```python
from build123d import *

# Parameters (mm, degrees)
BOSS_EXTRUDE1_DEPTH = 7.5
SKETCH2_R           = 6.1
BOSS_EXTRUDE2_DEPTH = 2.3
SKETCH3_R           = 7.625
BOSS_EXTRUDE3_DEPTH = 1.3
CUT_EXTRUDE1_DEPTH  = 12.1
CUT_EXTRUDE2_REACH  = 15.91
SKETCH5_R           = 1.5


with BuildPart() as part:
    # Sketch1 → Boss-Extrude1 (new body)
    with BuildSketch(Plane(origin=(0, 0, 0), x_dir=(1, 0, 0), z_dir=(0, 1, 0))):
        Polygon((7.257292884, 0), (3.628646442, 6.285), (-3.628646442, 6.285), (-7.257292884, 0), (-3.628646442, -6.285), (3.628646442, -6.285), align=None)
    extrude(amount=BOSS_EXTRUDE1_DEPTH)

    # Sketch2 → Boss-Extrude2 (add)
    with BuildSketch(Plane(origin=(0, 7.5, 0), x_dir=(1, 0, 0), z_dir=(0, 1, 0))):
        Circle(SKETCH2_R)
    extrude(amount=BOSS_EXTRUDE2_DEPTH)

    # Sketch3 → Boss-Extrude3 (add)
    with BuildSketch(Plane.XZ):
        Circle(SKETCH3_R)
    extrude(amount=BOSS_EXTRUDE3_DEPTH)

    # Sketch4 → Cut-Extrude1 (cut, through all)
    with BuildSketch(Plane(origin=(0, 9.8, 0), x_dir=(1, 0, 0), z_dir=(0, 1, 0))):
        with BuildLine():
            Line((-1.12, -0.997797575), (1.12, -0.997797575))
            ThreePointArc((1.12, -0.997797575), (0, 1.5), (-1.12, -0.997797575))
        make_face()
    extrude(amount=-CUT_EXTRUDE1_DEPTH, mode=Mode.SUBTRACT)

    # Sketch5 → Cut-Extrude2 (cut, up to next)
    with BuildSketch(Plane.XY.offset(6.285), mode=Mode.PRIVATE) as cut_extrude2_sk1:
        with Locations((0, 3.75)):
            Circle(SKETCH5_R)
    cut_extrude2_tool1 = extrude(cut_extrude2_sk1.sketch, amount=-CUT_EXTRUDE2_REACH, mode=Mode.PRIVATE) & part.part
    add(cut_extrude2_tool1.solids().sort_by_distance((0, 3.75, 6.285))[0], mode=Mode.SUBTRACT)


solid = part.part
```
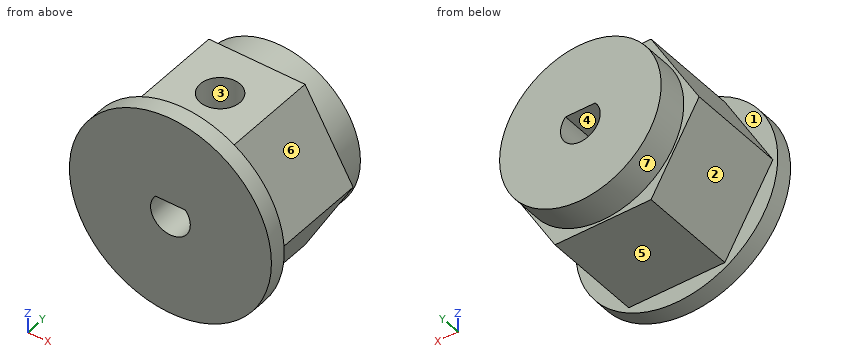
Check sheet for the modelled part. Datum: model origin and axes. Units: mm. Face numbers are marked on the shaded views. A direction names the side the tool comes from. Coordinates: 2 decimals unless noted, no trailing zeros. Order: outer loops, then holes, each group sorted by start corner. A loop starts at its lowest first (then second) coordinate and runs counter-clockwise, first axis right, second up. Notation, with made-up numbers: M -2,-36.75 L 3,-36.75 A14 ccw 3,-32.75 Z; hole C 60.25,-13.75 d6. An arc over 180 degrees is marked long. Write each question's results on one line, items separated by ' | '. Start each with the question number.
1. Cross-section at C-C on z = 1.5. Record the cut outline in (x, y), and give its area (3 significant figures).
2. Access from +Z, -Z, +X, -X, +Y, -Y to the whole of each face (thin tool, end or side, straight path). Record for the marked faces 4, 5, 6 and 7.
3. Mould release check, pull along Y, two halves, no side actions. Record for the marked faces 1, 2 and 3: +Y half, -Y half, draft (parallel to the pull), parting line (faces both ways), or undercut.
4. Cross-section at B-B on y = 6.5. Record the cut outline in (x, z) (3 decimals), and give its area (3 significant figures).
5. Material ranges on probe 1 along Z at (x, y) = (0, 5.5) (3 decimals); probe 2 along Z at (x, y) = (2, 1.25) (3 decimals); probe 3 along X at (y, z) = (3.75, 4), recorded low to high.
6. Go/stop test with flat-tipped pins: P1, Ø3.5, axis at x = -1.5, y = 4.5, coming from the +Z side (3 decimals); P2, Ø6, axis at x = -2.5, y = 8.5, coming from the -Z side (3 decimals); P3, Ø1.5, axis at x = 5, y = 4.5, coming from the -Z side. Record where each tip stops, or that it passes through.
7. Cross-section at D-D on y = 3.75. Record the cut outline in (x, z) (3 decimals).
8. Cross-section at A-A on x = 0. Record the cut outline in (y, z) (3 decimals).
Checks:
1) outline: M -7.48,-1.3 L 7.48,-1.3 L 7.48,0 L 6.39,0 L 6.39,7.5 L 5.91,7.5 L 5.91,9.8 L -5.91,9.8 L -5.91,7.5 L -6.39,7.5 L -6.39,0 L -7.48,0 Z; hole C 0,3.75 d3 | area: 135 mm²
2) face 4: +Y, -Y | face 5: -Z, +X, -X, +Y | face 6: +Z, +X, +Y | face 7: +Y
3) face 1: +Y half | face 2: draft | face 3: undercut
4) outline: M -7.257,0 L -3.629,-6.285 L 3.629,-6.285 L 7.257,0 L 3.629,6.285 L -3.629,6.285 Z; hole M -1.12,0.998 A1.5 ccw long 1.12,0.998 Z | area: 131 mm²
5) probe 1: z = -6.285 to -1.5, 0.998 to 6.285 | probe 2: z = -6.285 to 6.285 | probe 3: x = -4.95 to -1.5, 1.5 to 4.95
6) P1: stops at z = 6.285 | P2: stops at z = -6.285 | P3: stops at z = -5.21
7) outline: M -7.257,0 L -3.629,-6.285 L 3.629,-6.285 L 7.257,0 L 3.629,6.285 L 1.5,6.285 L 1.5,0 A1.5 cw -1.5,0 L -1.5,6.285 L -3.629,6.285 Z
8) outline: M -1.3,-7.625 L 0,-7.625 L 0,-6.285 L 7.5,-6.285 L 7.5,-6.1 L 9.8,-6.1 L 9.8,-1.5 L -1.3,-1.5 Z; M -1.3,0.998 L 2.25,0.998 L 2.25,6.285 L 0,6.285 L 0,7.625 L -1.3,7.625 Z; M 5.25,0.998 L 9.8,0.998 L 9.8,6.1 L 7.5,6.1 L 7.5,6.285 L 5.25,6.285 Z
